```python
from build123d import *

# Parameters (mm, degrees)
SKETCH_1_W          = 80
SKETCH_1_H          = 50
EXTRUDE_1_DEPTH     = 10
SKETCH_2_R          = 2.5
SKETCH_2_R_2        = 1.25
EXTRUDE_2_DEPTH     = 20
SKETCH_4_W          = 25
SKETCH_4_H          = 50
EXTRUDE_3_DEPTH     = 8
SKETCH_5_R          = 1.25
EXTRUDE_4_DEPTH     = 12
CUT_EXTRUDE_1_DEPTH = 77.576758876


with BuildPart() as part:
    # 草圖1 → 填料-伸長1 (new body)
    with BuildSketch(Plane(origin=(0, 0, 0), x_dir=(1, 0, 0), z_dir=(0, 1, 0))):
        Rectangle(SKETCH_1_W, SKETCH_1_H)
    extrude(amount=EXTRUDE_1_DEPTH)

    # 草圖2 → 填料-伸長2 (add)
    with BuildSketch(Plane(origin=(0, 10, 0), x_dir=(1, 0, 0), z_dir=(0, 1, 0))):
        with Locations(Location((-17.5, 0, 0), (0, 0, 270))):
            Circle(SKETCH_2_R)
        with Locations(Location((17.5, 0, 0), (0, 0, 270))):
            Circle(SKETCH_2_R_2)
    extrude(amount=EXTRUDE_2_DEPTH)

    # 草圖4 → 填料-伸長3 (add)
    with BuildSketch(Plane(origin=(0, 10, 0), x_dir=(1, 0, 0), z_dir=(0, 1, 0))):
        with Locations((27.5, 0)):
            Rectangle(SKETCH_4_W, SKETCH_4_H)
    extrude(amount=EXTRUDE_3_DEPTH)

    # 草圖5 → 填料-伸長4 (add)
    with BuildSketch(Plane(origin=(0, 30, 0), x_dir=(1, 0, 0), z_dir=(0, 1, 0))):
        with Locations(Location((17.5, 0, 0), (0, 0, 90))):
            Circle(SKETCH_5_R)
    extrude(amount=EXTRUDE_4_DEPTH)

    # 草圖7 → 除料-伸長1 (cut, through all)
    with BuildSketch(Plane(origin=(0, 0, -25), x_dir=(-1, 0, 0), z_dir=(0, 0, -1))):
        with BuildLine():
            Line((-15.473976981, 16), (-16.526023019, 16))
            ThreePointArc((-16.526023019, 16), (-16.861175356, 15.861175356), (-17, 15.526023019))
            Line((-17, 15.526023019), (-17, 10.473976981))
            ThreePointArc((-17, 10.473976981), (-16.861175356, 10.138824644), (-16.526023019, 10))
            Line((-16.526023019, 10), (-15, 10))
            Line((-15, 10), (-14.5, 10))
            Line((-14.5, 10), (-14.5, 18))
            Line((-14.5, 18), (-15, 18))
            Line((-15, 18), (-15, 16.473976981))
            ThreePointArc((-15, 16.473976981), (-15.138824644, 16.138824644), (-15.473976981, 16))
        make_face()
    extrude(amount=-CUT_EXTRUDE_1_DEPTH, mode=Mode.SUBTRACT)


solid = part.part
```
Geometry check sheet. Reference: the model listing, model coordinates, mm. A direction names the side the tool comes from. Round coordinates to 2 decimals unless told otherwise and drop trailing zeros. Write each loop counter-clockwise with the first axis right and the second up, starting at its lowest first coordinate (ties: lowest second). Pieces come first, ordered by that corner, then holes. Notation, with made-up numbers: (-23.5, 62.5) -> (22.5, 62.5) arc R34 ccw to (22.5, 99.5) -> close; hole circle Ø2 at (-38, -0.75). An arc over 180 degrees is marked (long way). Put each result on its own line as item: value.
1) Cross-section at A-A, the plane y = 14. Enter the section's corners in (x, z).
Recorded:
outline: circle Ø5 at (-17.5, 0); (17, -25) -> (40, -25) -> (40, 25) -> (17, 25) -> close
2) Access from +Z, -Z, +X, -X, +Y, -Y to the whole of each face (thin tool, end or side, straight path). Record for faces 1 (the face through (-17, 30, 0)), 2 (the face through (-1, 0, 0)).
Recorded:
face 1: +Z, -Z, -X, +Y
face 2: +Z, -Z, +X, -X, -Y
3) Depth check by flat-ended pin: P1, Ø3, axis at y = 17, z = -2.5, coming from the -X side; P2, Ø0.8, axis at x = 16, z = -10, coming from the +Y side; P3, Ø2.5, axis at y = 13.5, z = 2, coming from the -X side. Enter the tip coordinate at first touch or a pass-through.
Recorded:
P1: stops at x = -19.79
P2: stops at y = 18
P3: stops at x = -19.88
4) Cross-section at D-D, the plane y = 31. Enter the section's corners in (x, z), plus the area to 3 significant figures.
Recorded:
outline: circle Ø2.5 at (17.5, 0)
area: 4.91 mm2
5) Cross-section at B-B, the plane z = 0. Enter the section's corners in (x, y).
Recorded:
outline: (-40, 0) -> (40, 0) -> (40, 18) -> (18.75, 18) -> (18.75, 42) -> (16.25, 42) -> (16.25, 18) -> (15, 18) -> (15, 16.47) arc R0.47 ccw to (15.47, 16) -> (16.53, 16) arc R0.47 cw to (17, 15.53) -> (17, 10.47) arc R0.47 cw to (16.53, 10) -> (-15, 10) -> (-15, 30) -> (-20, 30) -> (-20, 10) -> (-40, 10) -> close
6) Thickness scan on probe 1 along Y at (x, z) = (4, -7); probe 2 along Y at (x, z) = (20.5, 13); probe 3 along X at (y, z) = (11.5, 9). Record the ranges inside material, lowest first. Write a range as from..to.
Recorded:
probe 1: y = 0..10
probe 2: y = 0..18
probe 3: x = 17..40
7) Release check for a two-part mould opening along X. For faces 3 (the face through (-40, 5, 0)), 4 (the face through (8, 7, 25)), 5 (the face through (-19.94, 19.86, -0.54)), 6 (the face through (40, 9, 0)) record: pulls with the +X half, pulls with the -X half, needs draft (parallel to the pull), parting line crosses it, or undercut.
Recorded:
face 3: pulls with the -X half
face 4: needs draft
face 5: undercut
face 6: pulls with the +X half
8) Cross-section at C-C, the plane x = -17.5. Enter the section's corners in (y, z).
Recorded:
outline: (0, -25) -> (10, -25) -> (10, -2.5) -> (30, -2.5) -> (30, 2.5) -> (10, 2.5) -> (10, 25) -> (0, 25) -> close
